Build history of the part. All positions in model axes, mm. A direction names the side the tool comes from. Give positions to 0.01 mm unless a question says otherwise; leave off trailing zeros. Use one line per item in the form item = value. Start each with the question number.
from build123d import *

# Parameters (mm, degrees)
SKETCH1_W           = 38.1
SKETCH1_H           = 609.6
BOSS_EXTRUDE1_DEPTH = 15.875
SKETCH2_R           = 4.7625
CUT_EXTRUDE1_DEPTH  = 308.581965702
SKETCH3_R           = 6.35
CUT_EXTRUDE2_DEPTH  = 19.431
CHAMFER1_SIZE       = 12.7
SKETCH4_R           = 16.1925
CUT_EXTRUDE3_DEPTH  = 1.778
SKETCH5_R           = 9.017
CUT_EXTRUDE4_DEPTH  = 1.524
SKETCH6_R           = 0.762
CUT_EXTRUDE5_DEPTH  = 12.7


with BuildPart() as part:
    # Sketch1 → Boss-Extrude1 (new body)
    with BuildSketch(Plane(origin=(0, 0, 0), x_dir=(0, 0, -1), z_dir=(1, 0, 0))):
        Rectangle(SKETCH1_W, SKETCH1_H)
    extrude(amount=BOSS_EXTRUDE1_DEPTH)

    # Sketch2 → Cut-Extrude1 (cut, through all)
    with BuildSketch(Plane.XY.offset(19.05)):
        with Locations((7.9375, -247.65)):
            Circle(SKETCH2_R)
    extrude(amount=-CUT_EXTRUDE1_DEPTH, mode=Mode.SUBTRACT)

    # Sketch3 → Cut-Extrude2 (cut)
    with BuildSketch(Plane.XY.offset(19.05)):
        with Locations((7.9375, -247.65)):
            Circle(SKETCH3_R)
    extrude(amount=-CUT_EXTRUDE2_DEPTH, mode=Mode.SUBTRACT)

    # Chamfer1
    chamfer1_edges = [part.edges().sort_by_distance(p)[0] for p in [
        (7.9375, -304.8, -19.05),
        (7.9375, -304.8, 19.05),
    ]]
    chamfer(chamfer1_edges, length=CHAMFER1_SIZE)

    # Sketch4 → Cut-Extrude3 (cut)
    with BuildSketch(Plane(origin=(0, 0, -19.05), x_dir=(-1, 0, 0), z_dir=(0, 0, -1))):
        with Locations((-7.9375, -247.65)):
            Circle(SKETCH4_R)
    extrude(amount=-CUT_EXTRUDE3_DEPTH, mode=Mode.SUBTRACT)

    # Sketch5 → Cut-Extrude4 (cut)
    with BuildSketch(Plane.XY.offset(19.05)):
        with Locations((7.9375, -247.65)):
            Circle(SKETCH5_R)
    extrude(amount=-CUT_EXTRUDE4_DEPTH, mode=Mode.SUBTRACT)

    # Sketch6 → Cut-Extrude5 (cut)
    with BuildSketch(Plane(origin=(0, 0, -17.272), x_dir=(-1, 0, 0), z_dir=(0, 0, -1))):
        with Locations(Location((-7.9375, -235.331, 0), (0, 0, 90))):
            Circle(SKETCH6_R)
    extrude(amount=-CUT_EXTRUDE5_DEPTH, mode=Mode.SUBTRACT)


solid = part.part
(1) Two-plate mould, pull along X, no slides. Class faces 4 (the cylindrical face through (6.9, -252.3, -8.7)), 5 (the flat face through (0, 4, 0)), 6 (the flat face through (7.83, -298.54, 12.61)): +X half, -X half, draft (parallel to the pull), parting line (faces both ways), or undercut.
(2) Pin check, flat tip, straight feed: pin 1 Ø1 at (x, z) = (8, 9) entering from -Y. Stop position of the tip, or through.
(3) Wall check: line 1 (Y direction, x = 7.25, z = -0.5); line 2 (X direction, y = -247, z = 4) (3 decimals); line 3 (X direction, y = -247, z = -13) (3 decimals). Give the ranges that are in metal, low to high. Write a range as from..to.
(4) Which spindle directions (+Z, -Z, +X, -X, +Y, -Y) get a long thin tool onto all of the face, cutting with end or side? Do faces 1 (the flat face through (12, -251, -17.272)), 2 (the flat face through (8, 304.8, 0)), 3 (the flat face through (10, -243, -0.381)). Say none if no direction does.
Solution:
q1.face_4 = undercut
q1.face_5 = -X half
q1.face_6 = draft
q2.pin_1 = -302.65
q3.line_1 = -304.8..-252.36, -242.94..304.8
q3.line_2 = 0..1.621, 14.254..15.875
q3.line_3 = 0..3.22, 12.655..15.875
q4.face_1 = -Z
q4.face_2 = +Z, -Z, +X, -X, +Y
q4.face_3 = +Z
